from build123d import *

# Parameters (mm, degrees)
BOSS_EXTRUDE1_DEPTH = 6
BOSS_EXTRUDE3_DEPTH = 15
SKETCH4_R           = 1.7
CUT_EXTRUDE1_DEPTH  = 10
CUT_EXTRUDE2_START  = -10
CUT_EXTRUDE2_DEPTH  = 4
SKETCH2_4_R         = 6.55
CUT_EXTRUDE3_DEPTH  = 5.1
SKETCH2_5_R         = 2.15
CUT_EXTRUDE4_DEPTH  = 68.88961629


with BuildPart() as part:
    # Sketch1 → Boss-Extrude1 (new body)
    with BuildSketch(Plane(origin=(0, 0, 0), x_dir=(1, 0, 0), z_dir=(0, 1, 0))):
        Polygon((0, 0), (60, 0), (60, 20), (37.5, 28), (22.5, 28), (0, 20), align=None)
    extrude(amount=BOSS_EXTRUDE1_DEPTH)

    # Sketch3 → Boss-Extrude3 (add)
    with BuildSketch(Plane(origin=(0, 6, 0), x_dir=(1, 0, 0), z_dir=(0, 1, 0))):
        Polygon((0, 10), (0, 0), (15, 0), (8.25, 4.5), align=None)
        Polygon((8.25, 4.5), (15, 0), (45, 0), (51.75, 4.5), align=None)
        Polygon((51.75, 4.5), (45, 0), (60, 0), (60, 10), align=None)
    extrude(amount=BOSS_EXTRUDE3_DEPTH)

    # Sketch4 → Cut-Extrude1 (cut)
    with BuildSketch(Plane(origin=(0, 21, 0), x_dir=(1, 0, 0), z_dir=(0, 1, 0))):
        with Locations(Location((3, 4.25, 0), (0, 0, 270))):
            Circle(SKETCH4_R)
        with Locations(Location((57, 4.25, 0), (0, 0, 270))):
            Circle(SKETCH4_R)
    extrude(amount=-CUT_EXTRUDE1_DEPTH, mode=Mode.SUBTRACT)

    # Sketch6 → Cut-Extrude2 (cut)
    with BuildSketch(Plane(origin=(0, 21, 0), x_dir=(1, 0, 0), z_dir=(0, 1, 0)).offset(CUT_EXTRUDE2_START)):
        Polygon((5.5, 0), (5.5, 2.806624327), (3, 1.363248654), (0.5, 2.806624327), (0.5, 0), align=None)
        Polygon((3, 1.363248654), (5.5, 2.806624327), (5.5, 5.693375673), (3, 7.136751346), (0.5, 5.693375673), (0.5, 2.806624327), align=None)
        Polygon((59.5, 5.693375673), (57, 7.136751346), (54.5, 5.693375673), (54.5, 2.806624327), (57, 1.363248654), (59.5, 2.806624327), align=None)
        Polygon((57, 1.363248654), (54.5, 2.806624327), (54.5, 0), (59.5, 0), (59.5, 2.806624327), align=None)
    extrude(amount=-CUT_EXTRUDE2_DEPTH, mode=Mode.SUBTRACT)

    # Sketch2_4 → Cut-Extrude3 (cut)
    with BuildSketch(Plane(origin=(0, 6, 0), x_dir=(1, 0, 0), z_dir=(0, 1, 0))):
        with Locations(Location((7.5, 13, 0), (0, 0, 270))):
            Circle(SKETCH2_4_R)
        with Locations(Location((22.5, 13, 0), (0, 0, 270))):
            Circle(SKETCH2_4_R)
        with Locations(Location((37.5, 13, 0), (0, 0, 270))):
            Circle(SKETCH2_4_R)
        with Locations(Location((52.5, 13, 0), (0, 0, 270))):
            Circle(SKETCH2_4_R)
    extrude(amount=-CUT_EXTRUDE3_DEPTH, mode=Mode.SUBTRACT)

    # Sketch2_5 → Cut-Extrude4 (cut, through all)
    with BuildSketch(Plane(origin=(0, 6, 0), x_dir=(1, 0, 0), z_dir=(0, 1, 0))):
        with Locations(Location((7.5, 13, 0), (0, 0, 270))):
            Circle(SKETCH2_5_R)
        with Locations(Location((22.5, 13, 0), (0, 0, 270))):
            Circle(SKETCH2_5_R)
        with Locations(Location((37.5, 13, 0), (0, 0, 270))):
            Circle(SKETCH2_5_R)
        with Locations(Location((52.5, 13, 0), (0, 0, 270))):
            Circle(SKETCH2_5_R)
    extrude(amount=-CUT_EXTRUDE4_DEPTH, mode=Mode.SUBTRACT)


solid = part.part
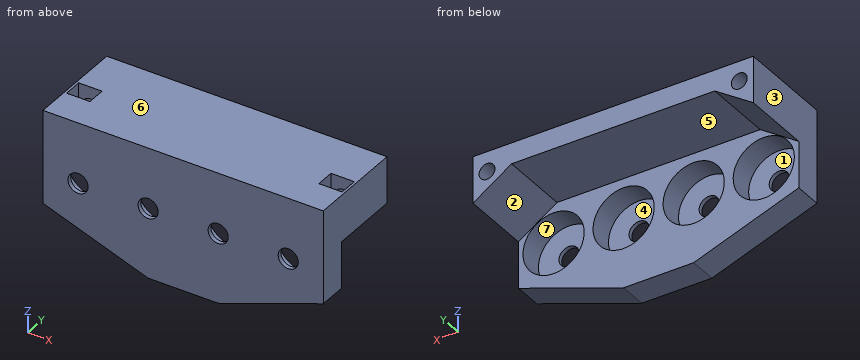
Could you check a few things on this model? Use its own coordinates, in mm. Face numbers are marked on the shaded views. A direction names the side the tool comes from. Round coordinates to 2 decimals unless told otherwise and drop trailing zeros. Write each loop counter-clockwise with the first axis right and the second up, starting at its lowest first coordinate (ties: lowest second). Pieces come first, ordered by that corner, then holes. Notation, with made-up numbers: (1, 25.5) -> (27, 25.5) arc R25 cw to (27, 57.5) -> close; hole circle Ø1 at (-39, -38.75). An arc over 180 degrees is marked (long way). Use a Markdown table: item, result.
1. Please list where these lines run through material, in increasing order: probe 1 along X at (y, z) = (0.5, -13); probe 2 along X at (y, z) = (3.1, -13); probe 3 along Y at (x, z) = (4, -5.75).
Answer key:
| item | result |
|---|---|
| probe 1 | x = 0 to 5.35, 9.65 to 20.35, 24.65 to 35.35, 39.65 to 50.35, 54.65 to 60 |
| probe 2 | x = 0 to 0.95, 14.05 to 15.95, 29.05 to 30.95, 44.05 to 45.95, 59.05 to 60 |
| probe 3 | y = 0 to 7, 11 to 21 |
2. For pin 1 Ø3 at (x, z) = (57, -4.25) entering from +Y; pin 2 Ø6 at (x, z) = (35.5, -15) entering from +Y; pin 3 Ø3.5 at (x, z) = (52.5, -13) entering from +Y; pin 4 Ø7.5 at (x, y) = (28.5, 13.5) entering from -Z, each with a flat end and sliding along its axis, tell me the tip position at first contact or that it passes through.
Answer key:
| item | result |
|---|---|
| pin 1 | stops at y = 7 |
| pin 2 | stops at y = 0.9 |
| pin 3 | passes through |
| pin 4 | stops at z = -4.5 |
3. If we section it at D-D (y = 9.75): List the corners of the cut face in (x, z) for me.
Answer key:
| item | result |
|---|---|
| outline | (0, -10) -> (8.25, -4.5) -> (51.75, -4.5) -> (60, -10) -> (60, 0) -> (59.5, 0) -> (59.5, -5.69) -> (57, -7.14) -> (54.5, -5.69) -> (54.5, 0) -> (5.5, 0) -> (5.5, -5.69) -> (3, -7.14) -> (0.5, -5.69) -> (0.5, 0) -> (0, 0) -> close |
4. Which directions (+Z, -Z, +X, -X, +Y, -Y) give clear straight access to the entire face, cutting with the end or side of a thin tool? Please do the marked faces 5, 6 and 7.
Answer key:
| item | result |
|---|---|
| face 5 | -Z, +Y |
| face 6 | +Z, +X, -X, +Y, -Y |
| face 7 | +Y |
5. If we section it at C-C (x = 30): List the corners of the cut face in (y, z) for me.
Answer key:
| item | result |
|---|---|
| outline | (0, -28) -> (6, -28) -> (6, -4.5) -> (21, -4.5) -> (21, 0) -> (0, 0) -> close |
6. If we section it at A-A (y = 13.25): List the corners of the cut face in (x, z) for me, then the cut area to 3 significant figures.
Answer key:
| item | result |
|---|---|
| outline | (0, -10) -> (8.25, -4.5) -> (51.75, -4.5) -> (60, -10) -> (60, 0) -> (0, 0) -> close; hole circle Ø3.4 at (3, -4.25); hole circle Ø3.4 at (57, -4.25) |
| area | 297 mm^2 |
7. If we section it at B-B (y = 2.75): List the corners of the cut face in (x, z) for me.
Answer key:
| item | result |
|---|---|
| outline | (0, -20) -> (22.5, -28) -> (37.5, -28) -> (60, -20) -> (60, 0) -> (0, 0) -> close; hole circle Ø13.1 at (7.5, -13); hole circle Ø13.1 at (22.5, -13); hole circle Ø13.1 at (37.5, -13); hole circle Ø13.1 at (52.5, -13) |
8. We'd pull the mould along Z, two halves only. Please class the marked faces 1, 2, 3 and 4: +Z half, -Z half, draft (parallel to the pull), parting line (faces both ways), or undercut.
Answer key:
| item | result |
|---|---|
| face 1 | undercut |
| face 2 | -Z half |
| face 3 | draft |
| face 4 | undercut |
